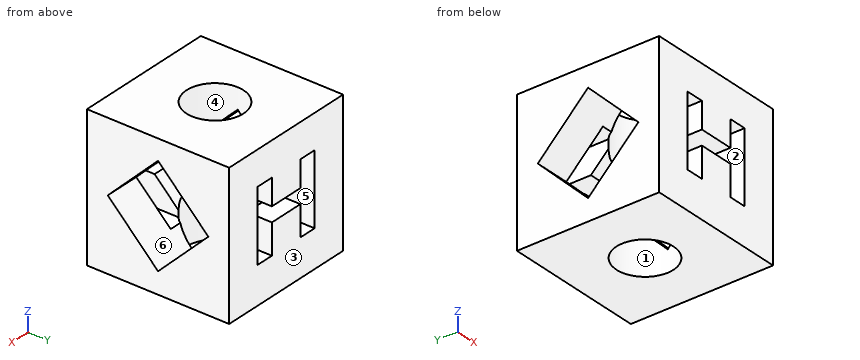
```python
from build123d import *

# Parameters (mm, degrees)
BOX_W           = 5
BOX_H           = 5
BOX_DEPTH       = 5
SKETCH_R        = 1
POCKET_DEPTH    = 7.5
POCKET001_DEPTH = 5
BOX001_W        = 2.5
BOX001_H        = 2.5
BOX001_DEPTH    = 5


with BuildPart() as part:
    # Box → Box (join)
    with BuildSketch(Plane.XY):
        with Locations((2.5, 2.5)):
            Rectangle(BOX_W, BOX_H)
    extrude(amount=BOX_DEPTH)

    # Sketch → Pocket (cut, symmetric)
    with BuildSketch(Plane.XY):
        with Locations((2.5, 2.5)):
            Circle(SKETCH_R)
    extrude(amount=POCKET_DEPTH, both=True, mode=Mode.SUBTRACT)

    # Sketch001 → Pocket001 (cut)
    with BuildSketch(Plane.XZ):
        Polygon((1.25, 3.806445), (1.25, 1.306445), (1.875, 1.306445), (1.875, 2.372529), (3.125, 2.372529), (3.125, 1.306445), (3.75, 1.306445), (3.75, 3.806445), (3.125, 3.806445), (3.125, 2.885704), (1.875, 2.885704), (1.875, 3.806445), align=None)
    extrude(amount=-POCKET001_DEPTH, mode=Mode.SUBTRACT)

    # Box001 → Box001 (cut)
    with BuildSketch(Plane(origin=(0, 2.5, 0.75), x_dir=(0, 0.707107, 0.707107), z_dir=(1, 0, 0))):
        with Locations((1.25, 1.25)):
            Rectangle(BOX001_W, BOX001_H)
    extrude(amount=BOX001_DEPTH, mode=Mode.SUBTRACT)


solid = part.part
```
CAD build for the part. Positions are in the model's coordinates, mm. Face numbers are marked on the shaded views. A direction names the side the tool comes from. Round coordinates to 2 decimals unless told otherwise and drop trailing zeros. Loops run counter-clockwise (first coordinate to the right, second up) from the corner with the lowest first, then second, coordinate; pieces in that order, holes last. Notation, with made-up numbers: M -36.5,61.25 L 1.5,61.25 A22 cw 1.5,99.25 Z; hole C 46,-12 d2. An arc over 180 degrees is marked long. Use a Markdown table: item, result. Add a question column.
(1) Cut at C-C (y = 3.8). Give the cut face in (x, z) (3 decimals).
(2) Pull direction Y, two halves, no side cores. Call the marked faces 1, 2 and 3: +Y half, -Y half, draft (parallel to the pull), parting line (faces both ways), or undercut.
(3) Cut at D-D (z = 4). Give the cut face in (x, y), and give its area (3 significant figures).
(4) Drill centre lines: line 1 (X direction, y = 1.1, z = 1.7) (3 decimals); line 2 (Y direction, x = 2.5, z = 0.6). Where is each one in solid material? Low to high.
(5) Cut at A-A (x = 2.5). Give the cut face in (y, z).
(6) Which spindle directions (+Z, -Z, +X, -X, +Y, -Y) get a long thin tool onto all of the face, cutting with end or side? Do the marked faces 4, 5 and 6. Say none if no direction does.
(7) Flat gauge pins, fed straight in: pin 1 (0.5 mm diameter, centred on y = 4, z = 2, fed in from -X); pin 2 (1.2 mm diameter, centred on x = 2.5, y = 2.5, fed in from -Z). Where does each tip first touch, or does it go through?
(8) Cut at B-B (z = 1.9). Give the cut face in (x, y) (3 decimals).
Geometry says:
| question | item | result |
|---|---|---|
| 1 | outline | M 0,0 L 5,0 L 5,2.05 L 3.75,2.05 L 3.75,1.306 L 3.125,1.306 L 3.125,2.05 L 1.875,2.05 L 1.875,1.306 L 1.25,1.306 L 1.25,2.05 L 0,2.05 Z; M 0,2.986 L 1.25,2.986 L 1.25,3.806 L 1.875,3.806 L 1.875,2.986 L 3.125,2.986 L 3.125,3.806 L 3.75,3.806 L 3.75,2.986 L 5,2.986 L 5,5 L 0,5 Z |
| 2 | face 1 | undercut |
| 2 | face 2 | draft |
| 2 | face 3 | +Y half |
| 3 | outline | M 0,0 L 5,0 L 5,2.21 L 3.46,2.21 A1 cw 1.54,2.21 L 0,2.21 Z; M 0,2.79 L 1.54,2.79 A1 cw 3.46,2.79 L 5,2.79 L 5,5 L 0,5 Z |
| 3 | area | 20.1 mm² |
| 4 | line 1 | x = 0 to 1.25, 1.875 to 3.125, 3.75 to 5 |
| 4 | line 2 | y = 0 to 1.5, 3.5 to 5 |
| 5 | outline | M 0,0 L 1.5,0 L 1.5,1.75 L 0.88,2.37 L 0,2.37 Z; M 0,2.89 L 1.1,2.89 L 1.5,3.29 L 1.5,5 L 0,5 Z; M 3.5,0 L 5,0 L 5,2.37 L 4.12,2.37 L 3.5,1.75 Z; M 3.5,3.29 L 3.9,2.89 L 5,2.89 L 5,5 L 3.5,5 Z |
| 6 | face 4 | +Z, -Z |
| 6 | face 5 | +Y, -Y |
| 6 | face 6 | +X, -X |
| 7 | pin 1 | stops at x = 0 |
| 7 | pin 2 | passes through |
| 8 | outline | M 0,0 L 1.25,0 L 1.25,1.35 L 0,1.35 Z; M 0,3.65 L 1.25,3.65 L 1.25,5 L 0,5 Z; M 1.875,0 L 3.125,0 L 3.125,1.35 L 1.875,1.35 Z; M 1.875,3.65 L 3.125,3.65 L 3.125,5 L 1.875,5 Z; M 3.75,0 L 5,0 L 5,1.35 L 3.75,1.35 Z; M 3.75,3.65 L 5,3.65 L 5,5 L 3.75,5 Z |
